Autodesk Inventor part; units mm, degrees
ref_plane "YZ Plane" through (0, 0, 0) normal (1, 0, 0) x (0, 1, 0)
ref_plane "XZ Plane" through (0, 0, 0) normal (0, 1, 0) x (-1, 0, 0)
ref_plane "XY Plane" through (0, 0, 0) normal (0, 0, 1) x (1, 0, 0)
sketch "Esboço1" plane through (0, 0, 0) normal (0, 1, 0) x (-1, 0, 0)
  circle A0 centre (89.65, -41.2701) radius 1.5
  circle A1 centre (89.65, -10.2701) radius 1.5
  circle A2 centre (14.65, -10.2701) radius 1.5
  circle A3 centre (14.65, -41.2701) radius 1.5
  line L0 (14.65, -10.2701) -> (10.65, -10.2701) construction
  line L1 (10.65, -10.2701) -> (10.65, -6.2701) construction
  line L2 (10.65, -6.2701) -> (93.65, -6.2701)
  line L3 (93.65, -6.2701) -> (93.65, -45.2701)
  line L4 (93.65, -45.2701) -> (10.65, -45.2701)
  line L5 (10.65, -45.2701) -> (10.65, -6.2701)
  line L6 (87.5, -38.8701) -> (87.5, -14.8701) construction
  line L7 (87.5, -14.8701) -> (16.5, -14.8701) construction
  line L8 (16.5, -14.8701) -> (16.5, -38.8701) construction
  line L9 (16.5, -38.8701) -> (87.5, -38.8701) construction
  line L10 (87.5, -14.8701) -> (88.5, -14.8701) construction
  line L11 (88.5, -14.8701) -> (88.5, -13.8701) construction
  line L12 (88.5, -13.8701) -> (87.5, -13.8701) construction
  line L13 (87.5, -13.8701) -> (87.5, -14.8701) construction
  circle A4 centre (14.65, -10.2701) radius 2.85
  circle A5 centre (14.65, -41.2701) radius 2.85
  circle A6 centre (89.65, -41.2701) radius 2.85
  circle A7 centre (89.65, -10.2701) radius 2.85
  line L14 (16.5, -14.8701) -> (87.5, -14.8701)
  line L15 (87.5, -14.8701) -> (87.5, -38.8701)
  line L16 (87.5, -38.8701) -> (16.5, -38.8701)
  line L17 (16.5, -38.8701) -> (16.5, -14.8701)
  point P0 (0, 0)
  dimension "d0" = 4
  dimension "d1" = 4
  dimension "d2" = 4
  dimension "d3" = 4
  dimension "d4" = 4
  dimension "d5" = 4
  dimension "d6" = 4
  dimension "d7" = 4
  dimension "d8" = 1
  dimension "d9" = 1
  dimension "d10" = 5.7
  dimension "d11" = 5.7
  dimension "d12" = 5.7
  dimension "d13" = 5.7
extrude "Extrusão1" add sketch "Esboço1" along normal blind 2.5 contours L2 L3 L4 L5
sketch "Esboço2" plane through (0, 2.5, 0) normal (0, 1, 0) x (1, 0, 0)
  line L0 (-93.65, 6.2701) -> (-10.65, 6.2701)
  line L1 (-93.65, 45.2701) -> (-93.65, 6.2701)
  line L2 (-10.65, 6.2701) -> (-93.65, 6.2701)
  line L3 (-93.65, 6.2701) -> (-93.65, 45.2701)
  line L4 (-93.65, 45.2701) -> (-10.65, 45.2701)
  line L5 (-10.65, 45.2701) -> (-10.65, 6.2701)
  line L6 (-87.5, 14.8701) -> (-87.5, 38.8701)
  line L7 (-16.5, 14.8701) -> (-87.5, 14.8701)
  line L8 (-87.5, 38.8701) -> (-16.5, 38.8701)
  line L9 (-16.5, 38.8701) -> (-16.5, 14.8701)
  line L10 (-16.5, 14.8701) -> (-87.5, 14.8701)
  line L11 (-87.5, 14.8701) -> (-87.5, 38.8701)
  point P0 (0, 0)
extrude "Extrusão2" add sketch "Esboço2" along normal blind 1
properties part number "painel lcd"
Design review of the part built by this model. Coordinates are the model's own, in mm. A direction names the side the tool comes from. Round coordinates to 2 decimals unless told otherwise and drop trailing zeros. Write each loop counter-clockwise with the first axis right and the second up, starting at its lowest first coordinate (ties: lowest second). Pieces come first, ordered by that corner, then holes.
Item 1: Draft analysis for pull direction X (two halves, no side actions). For faces 1 (the cylindrical face through (-87.549, 1.232, -43.196)), 2 (the flat face through (-93.65, 2, -25)), 3 (the flat face through (-52, 2, -6.27)), state which applies: released by +X, released by -X, zero draft, split by the parting line, or undercut.
Item 2: Consider section C-C on y = 0.75. Give the boundary of the cut face in (x, z).
Item 3: Wall thickness on L1, parallel to X at y = 2, z = -41.5; L2, parallel to X at y = 2.5, z = -36; L3, parallel to Z at x = -32, y = 3.1: over which ranges is each line inside the solid? List them lowest first.
Item 4: For faces 4 (the flat face through (-53, 2, -45.27)), 5 (the flat face through (-87.5, 2, -27)), 6 (the cylindrical face through (-16.182, 1.232, -43.673)), list the 3-axis set-ups (+Z, -Z, +X, -X, +Y, -Y) from which the entire face can be reached by the end or side of a thin tool; tool diameter is ignored.
Item 5: For pin 1 Ø6.5 at (x, z) = (-15.5, -11) entering from -Y; pin 2 Ø1.7 at (x, z) = (-90, -11) entering from -Y; pin 3 Ø8 at (x, z) = (-64.5, -31) entering from -Y, all flat-tipped, find the tip position at first contact; note any pin that passes through.
Item 6: Consider section B-B on x = -19.5. Give the boundary of the cut face in (y, z), and give its area (3 significant figures).
Item 7: Consider section D-D on z = -43. Give the boundary of the cut face in (x, y), and give its area (3 significant figures).
Item 8: Consider section A-A on z = -33. Give the boundary of the cut face in (x, y).
Check values:
1. face 1: undercut
1. face 2: released by -X
1. face 3: zero draft
2. outline: (-93.65, -45.27) - (-10.65, -45.27) - (-10.65, -6.27) - (-93.65, -6.27) - close; hole circle Ø5.7 at (-89.65, -41.27); hole circle Ø5.7 at (-89.65, -10.27); hole (-87.5, -38.87) - (-16.5, -38.87) - (-16.5, -14.87) - (-87.5, -14.87) - close; hole circle Ø5.7 at (-14.65, -41.27); hole circle Ø5.7 at (-14.65, -10.27)
3. L1: x = -93.65 to -92.49, -86.81 to -17.49, -11.81 to -10.65
3. L2: x = -93.65 to -87.5, -16.5 to -10.65
3. L3: z = -45.27 to -38.87, -14.87 to -6.27
4. face 4: -Z, +X, -X, +Y, -Y
4. face 5: +Y, -Y
4. face 6: -Y
5. pin 1: stops at y = 0
5. pin 2: stops at y = 2.5
5. pin 3: passes through
6. outline: (0, -45.27) - (3.5, -45.27) - (3.5, -38.87) - (0, -38.87) - close; (0, -14.87) - (3.5, -14.87) - (3.5, -6.27) - (0, -6.27) - close
6. area: 52.5 mm2
7. outline: (-93.65, 0) - (-91.91, 0) - (-91.91, 2.5) - (-87.39, 2.5) - (-87.39, 0) - (-16.91, 0) - (-16.91, 2.5) - (-12.39, 2.5) - (-12.39, 0) - (-10.65, 0) - (-10.65, 3.5) - (-93.65, 3.5) - close
7. area: 268 mm2
8. outline: (-93.65, 0) - (-87.5, 0) - (-87.5, 3.5) - (-93.65, 3.5) - close; (-16.5, 0) - (-10.65, 0) - (-10.65, 3.5) - (-16.5, 3.5) - close
